Read the model definition and answer for the solid it produces. Units are mm, in the model's axes. A direction names the side the tool comes from. Coordinates: 2 decimals unless noted, no trailing zeros. Write each loop counter-clockwise with the first axis right and the second up, starting at its lowest first coordinate (ties: lowest second). Pieces come first, ordered by that corner, then holes. Notation, with made-up numbers: (3.5, 73) - (26.5, 73) arc R18 ccw to (26.5, 90) - close; hole circle Ø11 at (-9.75, 45). An arc over 180 degrees is marked (long way). Return JSON: item names as keys, results as strings.
```python
from build123d import *

# Parameters (mm, degrees)
SKETCH1_R           = 41
BOSS_EXTRUDE1_DEPTH = 5
SKETCH2_R           = 2.5
BOSS_EXTRUDE2_DEPTH = 15
BOSS_EXTRUDE3_DEPTH = 40


with BuildPart() as part:
    # Sketch1 → Boss-Extrude1 (new body)
    with BuildSketch(Plane(origin=(0, 0, 0), x_dir=(1, 0, 0), z_dir=(0, 1, 0))):
        with Locations(Location((0, 0, 0), (0, 0, 270))):
            Circle(SKETCH1_R)
    extrude(amount=BOSS_EXTRUDE1_DEPTH)

    # Sketch2 → Boss-Extrude2 (add)
    with BuildSketch(Plane.XZ):
        with Locations(Location((28.730078072, 0, 0), (0, 0, 90))):
            Circle(SKETCH2_R)
        with Locations(Location((-14.365, 24.881, 0), (0, 0, 90))):
            Circle(SKETCH2_R)
        with Locations(Location((-14.365, -24.881, 0), (0, 0, 90))):
            Circle(SKETCH2_R)
    extrude(amount=BOSS_EXTRUDE2_DEPTH)

    # Sketch3 → Boss-Extrude3 (add)
    with BuildSketch(Plane(origin=(0, 5, 0), x_dir=(1, 0, 0), z_dir=(0, 1, 0))):
        with BuildLine():
            Line((-10, 31.356159261), (-10, -31.356159261))
            ThreePointArc((-10, -31.356159261), (-32.912136418, 0), (-10, 31.356159261))
        make_face()
        with BuildLine():
            Line((10, 31.356159261), (10, -31.356159261))
            ThreePointArc((10, -31.356159261), (32.912136418, 0), (10, 31.356159261))
        make_face()
    extrude(amount=BOSS_EXTRUDE3_DEPTH)


solid = part.part
```
(1) A cutting plane is placed at C-C (x = -27). Determine the outline of the cut face in (y, z), and give its area (3 significant figures).
Answer:
{"outline": "(0, -30.85) - (5, -30.85) - (5, -18.82) - (45, -18.82) - (45, 18.82) - (5, 18.82) - (5, 30.85) - (0, 30.85) - close", "area": "1,810 mm²"}
(2) Straight lines are drawn through the part: line 1 (Y direction, x = -31, z = -24); line 2 (X direction, y = 11.5, z = -7.5); line 3 (Y direction, x = 22.5, z = 4). For each, find the intervals that lie inside material, in ascending order. Write a range as from..to.
Answer:
{"line 1": "0..5", "line 2": "-32.05..-10, 10..32.05", "line 3": "0..45"}
(3) A cutting plane is placed at A-A (z = 0). Determine the outline of the cut face in (x, y), and give its area (3 significant figures).
Answer:
{"outline": "(-41, 0) - (26.23, 0) - (26.23, -15) - (31.23, -15) - (31.23, 0) - (41, 0) - (41, 5) - (32.91, 5) - (32.91, 45) - (10, 45) - (10, 5) - (-10, 5) - (-10, 45) - (-32.91, 45) - (-32.91, 5) - (-41, 5) - close", "area": "2,320 mm²"}
(4) A cutting plane is placed at D-D (x = 0). Determine the outline of the cut face in (y, z), and give its area (3 significant figures).
Answer:
{"outline": "(0, -41) - (5, -41) - (5, 41) - (0, 41) - close", "area": "410 mm²"}
(5) Flat-ended cylindrical pins translate along their axes: P1, Ø12, axis at x = 22.5, z = -25.5, coming from the -Y side; P2, Ø2, axis at x = -13, y = 31.5, coming from the +Z side; P3, Ø12, axis at y = 14, z = -9.5, coming from the +X side. Find the tip coordinate at first contact, or state that the pin passes through.
Answer:
{"P1": "y = 0", "P2": "z = 30.65", "P3": "x = 32.73"}
(6) Which of the six approach directions +Z, -Z, +X, -X, +Y, -Y give full straight-line access (tool end or side, diameter ignored) to faces 5 (the face through (-15.116, -7.395, 27.266)), 6 (the face through (-14, -15, -25)), 7 (the face through (-32.907, 24.72, 0.581)), 8 (the face through (32.907, 24.72, 0.581))?
Answer:
{"face 5": "-Y", "face 6": "+Z, -Z, +X, -X, -Y", "face 7": "-X, +Y", "face 8": "+X, +Y"}
(7) A cutting plane is placed at B-B (y = 25.5). Determine the outline of the cut face in (x, z), and give its area (3 significant figures).
Answer:
{"outline": "(-10, -31.36) - (-10, 31.36) arc R32.91 ccw to start; (10, -31.36) arc R32.91 ccw to (10, 31.36) - close", "area": "2,110 mm²"}
(8) Determine the mould class of faces 1 (the face through (31.17, -7.4, -0.54)), 2 (the face through (-10, 25, 0)), 3 (the face through (19, 45, 0)), 4 (the face through (10, 25, 0)) for opening direction X: +X half, -X half, draft (parallel to the pull), parting line (faces both ways), or undercut.
Answer:
{"face 1": "parting line", "face 2": "undercut", "face 3": "draft", "face 4": "undercut"}
